Build history of the part. All positions in model axes, mm. A direction names the side the tool comes from. Coordinates: 2 decimals unless noted, no trailing zeros. Loops run counter-clockwise (first coordinate to the right, second up) from the corner with the lowest first, then second, coordinate; pieces in that order, holes last.
(1) Two-plate mould, pull along Y, no slides. Class faces 3 (the face through (81.96, 442.89, 4.06)), 4 (the face through (-1, 233, 0)), 5 (the face through (43, 368, 3.6)): pulls with the +Y half, pulls with the -Y half, needs draft (parallel to the pull), parting line crosses it, or undercut.
(2) Slice it at B-B (x = -15). Give the cut face in (y, z), and give its area (3 significant figures).
(3) Flat gauge pins, fed straight in: P1, Ø4, axis at x = -1, y = 328, coming from the +Z side; P2, Ø2.5, axis at x = -29.34, y = 399.34, coming from the +Z side. Where does each tip first touch, or does it go through?
(4) Slice it at A-A (y = 89). Give the cut face in (x, z), and give its area (3 significant figures).
(5) Tool access for faces 1 (the face through (73.926, 50.628, 3.944)), 2 (the face through (1.846, 407.951, 5.831)): list every direction of +Z, -Z, +X, -X, +Y, -Y with a clear straight run to the whole face (end or side of a thin tool).
(6) Slice it at D-D (z = 2). Give the number of separate pieces and of enclosed holes in the cut face, and give its area (3 significant figures).
(7) Wall check: L1, parallel to Y at x = 0, z = 5.7; L2, parallel to Y at x = 0, z = 1.8; L3, parallel to X at y = 368.5, z = 6.25. Give the ranges that are in metal, low to high.
(8) Slice it at C-C (y = 355.5). Give the cut face in (x, z).
from build123d import *

# Parameters (mm, degrees)
SKETCH_1_W          = 200
SKETCH_1_H          = 460
EXTRUDE_1_DEPTH     = 8
SKETCH_2_R          = 30
CUT_EXTRUDE_1_DEPTH = 10
SKETCH_3_R          = 2.25
CUT_EXTRUDE_2_DEPTH = 10
SKETCH_4_R          = 4
CUT_EXTRUDE_3_DEPTH = 4.4
FILLET_1_R          = 60
SKETCH_5_R          = 4.25
CUT_EXTRUDE_4_DEPTH = 10


with BuildPart() as part:
    # 草图1 → 凸台-拉伸1 (new body)
    with BuildSketch(Plane.XY):
        with Locations((0, 230)):
            Rectangle(SKETCH_1_W, SKETCH_1_H)
    extrude(amount=EXTRUDE_1_DEPTH)

    # 草图2 → 切除-拉伸1 (cut)
    with BuildSketch(Plane(origin=(0, 0, 0), x_dir=(-1, 0, 0), z_dir=(0, 0, -1))):
        with Locations((0, 370)):
            Circle(SKETCH_2_R)
    extrude(amount=-CUT_EXTRUDE_1_DEPTH, mode=Mode.SUBTRACT)

    # 草图3 → 切除-拉伸2 (cut)
    with BuildSketch(Plane(origin=(0, 0, 0), x_dir=(-1, 0, 0), z_dir=(0, 0, -1))):
        with Locations((0, 411.5)):
            Circle(SKETCH_3_R)
        with Locations((29.344931419, 399.344931419)):
            Circle(SKETCH_3_R)
        with Locations((41.5, 370)):
            Circle(SKETCH_3_R)
        with Locations((29.344931419, 340.655068581)):
            Circle(SKETCH_3_R)
        with Locations((0, 328.5)):
            Circle(SKETCH_3_R)
        with Locations((-29.344931419, 340.655068581)):
            Circle(SKETCH_3_R)
        with Locations((-41.5, 370)):
            Circle(SKETCH_3_R)
        with Locations((-29.344931419, 399.344931419)):
            Circle(SKETCH_3_R)
    extrude(amount=-CUT_EXTRUDE_2_DEPTH, mode=Mode.SUBTRACT)

    # 草图4 → 切除-拉伸3 (cut)
    with BuildSketch(Plane.XY.offset(8)):
        with Locations((29.344931419, 399.344931419)):
            Circle(SKETCH_4_R)
        with Locations((41.5, 370)):
            Circle(SKETCH_4_R)
        with Locations((29.344931419, 340.655068581)):
            Circle(SKETCH_4_R)
        with Locations((0, 328.5)):
            Circle(SKETCH_4_R)
        with Locations((-29.344931419, 340.655068581)):
            Circle(SKETCH_4_R)
        with Locations((-41.5, 370)):
            Circle(SKETCH_4_R)
        with Locations((-29.344931419, 399.344931419)):
            Circle(SKETCH_4_R)
        with Locations((0, 411.5)):
            Circle(SKETCH_4_R)
    extrude(amount=-CUT_EXTRUDE_3_DEPTH, mode=Mode.SUBTRACT)

    # 圆角1
    fillet_1_edges = [part.edges().sort_by_distance(p)[0] for p in [
        (100, 460, 4),
        (-100, 460, 4),
    ]]
    fillet(fillet_1_edges, radius=FILLET_1_R)

    # 草图5 → 切除-拉伸4 (cut)
    with BuildSketch(Plane(origin=(0, 0, 0), x_dir=(-1, 0, 0), z_dir=(0, 0, -1))):
        with Locations((40, 49)):
            Circle(SKETCH_5_R)
        with Locations((70, 49)):
            Circle(SKETCH_5_R)
        with Locations((40, 89)):
            Circle(SKETCH_5_R)
        with Locations((70, 89)):
            Circle(SKETCH_5_R)
        with Locations((40, 217)):
            Circle(SKETCH_5_R)
        with Locations((40, 177)):
            Circle(SKETCH_5_R)
        with Locations((70, 177)):
            Circle(SKETCH_5_R)
        with Locations((70, 217)):
            Circle(SKETCH_5_R)
        with Locations(Location((-70, 217, 0), (0, 0, 180))):
            Circle(SKETCH_5_R)
        with Locations(Location((-70, 177, 0), (0, 0, 180))):
            Circle(SKETCH_5_R)
        with Locations(Location((-40, 177, 0), (0, 0, 180))):
            Circle(SKETCH_5_R)
        with Locations(Location((-40, 217, 0), (0, 0, 180))):
            Circle(SKETCH_5_R)
        with Locations(Location((-70, 89, 0), (0, 0, 180))):
            Circle(SKETCH_5_R)
        with Locations(Location((-40, 89, 0), (0, 0, 180))):
            Circle(SKETCH_5_R)
        with Locations(Location((-70, 49, 0), (0, 0, 180))):
            Circle(SKETCH_5_R)
        with Locations(Location((-40, 49, 0), (0, 0, 180))):
            Circle(SKETCH_5_R)
    extrude(amount=-CUT_EXTRUDE_4_DEPTH, mode=Mode.SUBTRACT)


solid = part.part
Response values:
1. face 3: pulls with the +Y half
1. face 4: needs draft
1. face 5: undercut
2. outline: (0, 0) - (344.02, 0) - (344.02, 8) - (0, 8) - close; (395.98, 0) - (460, 0) - (460, 8) - (395.98, 8) - close
2. area: 3,260 mm2
3. P1: stops at z = 3.6
3. P2: passes through
4. outline: (-100, 0) - (-74.25, 0) - (-74.25, 8) - (-100, 8) - close; (-65.75, 0) - (-44.25, 0) - (-44.25, 8) - (-65.75, 8) - close; (-35.75, 0) - (35.75, 0) - (35.75, 8) - (-35.75, 8) - close; (44.25, 0) - (65.75, 0) - (65.75, 8) - (44.25, 8) - close; (74.25, 0) - (100, 0) - (100, 8) - (74.25, 8) - close
4. area: 1,330 mm2
5. face 1: +Z, -Z
5. face 2: +Z
6. separate pieces: 1
6. enclosed holes: 25
6. area: 86,600 mm2
7. L1: y = 0 to 324.5, 332.5 to 340, 400 to 407.5, 415.5 to 460
7. L2: y = 0 to 326.25, 330.75 to 340, 400 to 409.25, 413.75 to 460
7. L3: x = -100 to -45.21, -37.79 to -29.96, 29.96 to 37.79, 45.21 to 100
8. outline: (-100, 0) - (-26.26, 0) - (-26.26, 8) - (-100, 8) - close; (26.26, 0) - (100, 0) - (100, 8) - (26.26, 8) - close
